Here's the drawing with two shaded views (mm, measured from the low corner). I have some questions. A direction names the side the tool comes from. Give positions to 0.01 mm unless a question says otherwise; leave off trailing zeros. Write each loop counter-clockwise with the first axis right and the second up, starting at its lowest first coordinate (ties: lowest second). Pieces come first, ordered by that corner, then holes.
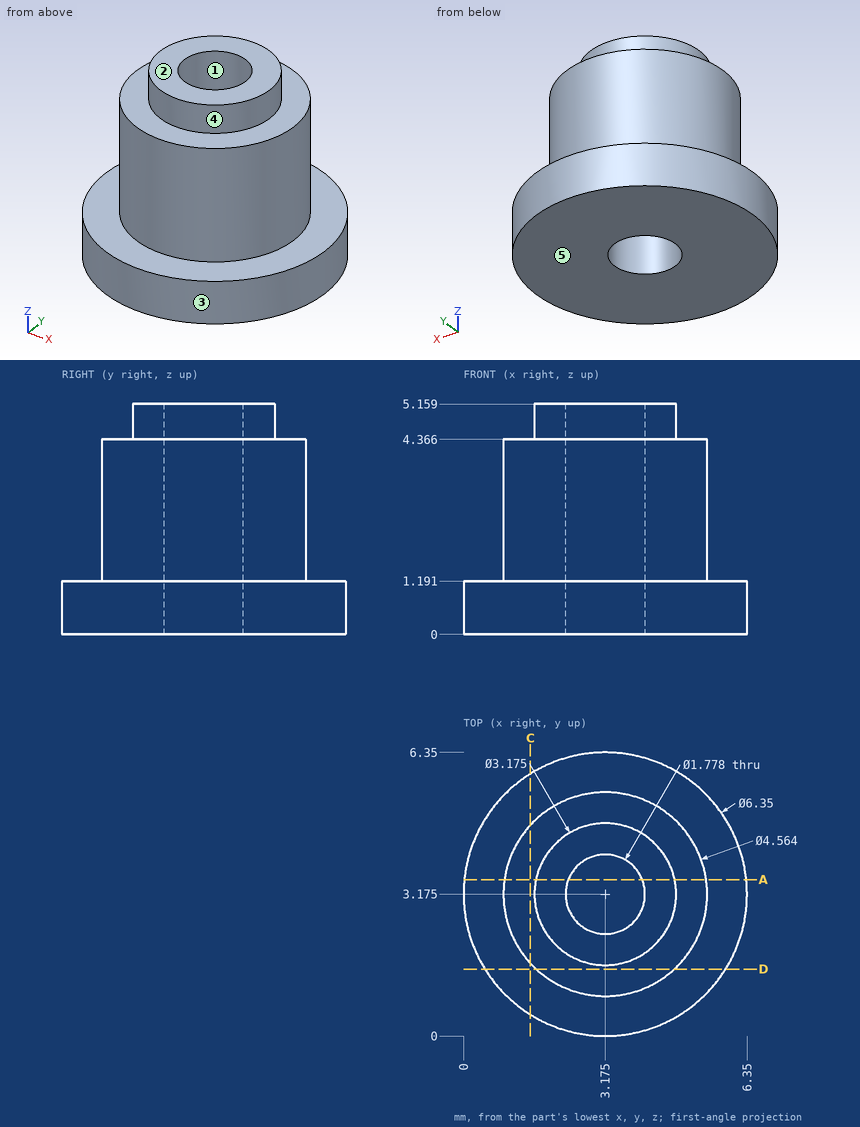
(1) Imagine slicing it at C-C, the plane x = 1.5. Write out the boundary of the cut face in (y, z) (1 decimal).
Returned:
outline: (0.5, 0) - (5.9, 0) - (5.9, 1.2) - (4.7, 1.2) - (4.7, 4.4) - (1.6, 4.4) - (1.6, 1.2) - (0.5, 1.2) - close
(2) For the marked faces 4 and 5, which set-ups out of +Z, -Z, +X, -X, +Y, -Y let a thin tool reach every point of the face, with its end or its side?
Returned:
face 4: +Z
face 5: -Z, +X, -X, +Y, -Y
(3) If I drill on L1, parallel to Z at x = 5, y = 5; L2, parallel to X at y = 3.75, z = 0.8 (1 decimal); L3, parallel to Z at x = 3.5, y = 1 (1 decimal), over which ranges is the centre line in solid material (lowest first)?
Returned:
L1: z = 0 to 1.19
L2: x = 0.1 to 2.5, 3.9 to 6.3
L3: z = 0 to 4.4
(4) Imagine slicing it at A-A, the plane y = 3.5. Write out the boundary of the cut face in (x, z) (1 decimal).
Returned:
outline: (0, 0) - (2.3, 0) - (2.3, 5.2) - (1.6, 5.2) - (1.6, 4.4) - (0.9, 4.4) - (0.9, 1.2) - (0, 1.2) - close; (4, 0) - (6.3, 0) - (6.3, 1.2) - (5.4, 1.2) - (5.4, 4.4) - (4.7, 4.4) - (4.7, 5.2) - (4, 5.2) - close
(5) Will these pins go through, and if not, where does the flat tip stop? P1, Ø2, axis at y = 1.5, z = 4.5, coming from the +X side; P2, Ø3, axis at y = 5.5, z = 1, coming from the -X side.
Returned:
P1: stops at x = 5.35
P2: stops at x = 0.11
(6) If we mould it in two halves opening along Y, with no side actions, what happens to the marked faces 1, 2 and 3? For each: +Y half, -Y half, draft (parallel to the pull), parting line (faces both ways), or undercut.
Returned:
face 1: undercut
face 2: draft
face 3: parting line
